```python
from build123d import *

# Parameters (mm, degrees)
F1_DEPTH = 20
F2_R     = 15
F3_DEPTH = 10
F3_TAPER = 5
F4_SIZE  = 2


with BuildPart() as f1:
    # F0 (on Front) → F1 (new body)
    with BuildSketch(Plane.XZ):
        with BuildLine():
            Line((0, -50), (105.8972473589, -24.2944947177))
            ThreePointArc((105.8972473589, -24.2944947177), (125, 0), (105.8972473589, 24.2944947177))
            Line((105.8972473589, 24.2944947177), (0, 50))
            Line((0, 50), (-50, 50))
            Line((-50, 50), (-50, -50))
            Line((-50, -50), (0, -50))
        make_face()
    extrude(amount=F1_DEPTH)

    # F2 (on face) → F3 (join)
    with BuildSketch(Plane.XZ.offset(20)):
        with Locations((100, 0)):
            Circle(F2_R)
    extrude(amount=F3_DEPTH, taper=F3_TAPER)

    # F4
    f4_edges = [f1.edges().sort_by_distance(p)[0] for p in [
        (52.948624, -20, 37.147247),
        (-25, -20, 50),
        (-50, -20, 0),
        (-25, -20, -50),
        (52.948624, -20, -37.147247),
        (125, -20, 0),
    ]]
    chamfer(f4_edges, length=F4_SIZE)


solid = f1.part
```
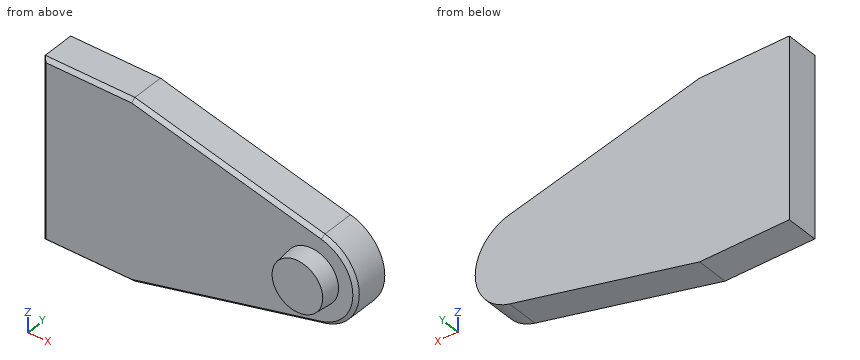
The model under review builds one solid part; all positions refer to its coordinate system, in mm. Round coordinates to 2 decimals unless told otherwise and drop trailing zeros. Loops run counter-clockwise (first coordinate to the right, second up) from the corner with the lowest first, then second, coordinate; pieces in that order, holes last. Notation, with made-up numbers: (32, 61.25) -> (90, 61.25) arc R19 cw to (90, 79.25) -> close; hole circle Ø6 at (5.5, 67.25). An arc over 180 degrees is marked (long way). Answer as a JSON object with one key per item and string values. Group by question number.
1) For pin 1 Ø3 at (x, z) = (4, 29) entering from -Y; pin 2 Ø10 at (y, z) = (-20.5, 21.5) entering from +X, all flat-tipped, find the tip position at first contact; note any pin that passes through.
2) For line 1 (Y direction, x = -17, z = -13.5); line 2 (X direction, y = -15, z = 0.5) (3 decimals); line 3 (Z direction, x = 0.5, y = -13.5), list the stretches that pass through material, from the lowest coordinate up. Write a range as [from, to].
3) We need section D-D on y = -24.5. Write out the cut boundary in (x, z), then the cut area to 3 significant figures.
4) We need section A-A on x = 100. Write out the cut boundary in (y, z).
5) We need section C-C on z = -26. Write out the cut boundary in (x, y).
6) We need section B-B on y = -7.5. Write out the cut boundary in (x, z).
Result set:
{
 "1": {"pin 1": "y = -20", "pin 2": "x = 118.17"},
 "2": {"line 1": "[-20, 0]", "line 2": "[-50, 124.995]", "line 3": "[-49.88, 49.88]"},
 "3": {"outline": "circle Ø29.21 at (100, 0)", "area": "670 mm²"},
 "4": {"outline": "(-30, -14.13) -> (-20, -15) -> (-20, -23.67) -> (-18, -25.73) -> (0, -25.73) -> (0, 25.73) -> (-18, 25.73) -> (-20, 23.67) -> (-20, 15) -> (-30, 14.13) -> close"},
 "5": {"outline": "(-50, -18) -> (-48, -20) -> (90.39, -20) -> (98.87, -18) -> (98.87, 0) -> (-50, 0) -> close"},
 "6": {"outline": "(-50, -50) -> (0, -50) -> (105.9, -24.29) arc R25 ccw to (105.9, 24.29) -> (0, 50) -> (-50, 50) -> close"}
}
